from build123d import *

# Parameters (mm, degrees)
SKETCH001_R      = 5
EXTRUDE001_DEPTH = 4
SKETCH_R         = 12.3
EXTRUDE_DEPTH    = 5
BOX001_W         = 82
BOX001_H         = 58
BOX001_DEPTH     = 44.4
BOX_W            = 74.7
BOX_H            = 38.74
BOX_DEPTH        = 44.4


with BuildPart() as extrude001:
    # Sketch001 (on Face3 of Extrude) → Extrude001 (new body)
    with BuildSketch(Plane.XY.offset(49.4)):
        with Locations((-58.7, 20.37)):
            Circle(SKETCH001_R)
    extrude(amount=EXTRUDE001_DEPTH)


with BuildPart() as extrude_body:
    # Sketch (on Face6 of Box001) → Extrude (new body)
    with BuildSketch(Plane(origin=(-82, -9.63, 44.4), x_dir=(1, 0, 0), z_dir=(0, 0, 1))):
        with Locations((23.3, 30)):
            Circle(SKETCH_R)
    extrude(amount=EXTRUDE_DEPTH)


with BuildPart() as cube001:
    # Box001 → Box001 (new body)
    with BuildSketch(Plane(origin=(-82, -9.63, 0), x_dir=(1, 0, 0), z_dir=(0, 0, 1))):
        with Locations((41, 29)):
            Rectangle(BOX001_W, BOX001_H)
    extrude(amount=BOX001_DEPTH)


with BuildPart() as fusion003:
    # Box → Box (new body)
    with BuildSketch(Plane.XY):
        with Locations((37.35, 19.37)):
            Rectangle(BOX_W, BOX_H)
    extrude(amount=BOX_DEPTH)

    # Fusion: union Cube001
    add(cube001.part)

    # Fusion002: union Extrude body
    add(extrude_body.part)

    # Fusion003: union Extrude001
    add(extrude001.part)


solid = fusion003.part
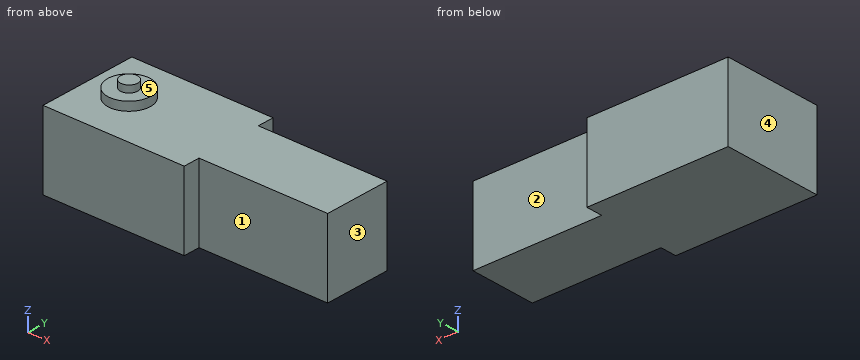
For this review, take the finished solid that the model builds, in its own axes (mm). Face numbers are marked on the shaded views. A direction names the side the tool comes from. Give positions to 0.01 mm unless a question says otherwise; leave off trailing zeros. Loops run counter-clockwise (first coordinate to the right, second up) from the corner with the lowest first, then second, coordinate; pieces in that order, holes last. Notation, with made-up numbers: M 38.5,73 L 89.5,73 A24 cw 89.5,87 Z; hole C 14.5,37.5 d2. An arc over 180 degrees is marked long. Answer as a JSON object with one key per item and string values. Group by question number.
Q1. Tool access review of the marked faces 1, 2, 3, 4 and 5: name each direction out of +Z, -Z, +X, -X, +Y, -Y from which nothing blocks a thin tool from reaching the whole face with its end or side.
Q2. Insertion check: P1, Ø17.5, axis at x = -10, y = 22.5, coming from the +Z side; P2, Ø8, axis at x = 49.5, z = 21, coming from the +Y side; P3, Ø1, axis at x = 18, z = 9.5, coming from the -Y side. Each pin has a flat end and moves straight along its axis. Give the tip position at first contact, or say it passes through.
Q3. Add section B-B on y = 20.37. Give the boundary of the cut face in (x, z).
Q4. Add section C-C on z = 4. Give the boundary of the cut face in (x, y), and give its area (3 significant figures).
Q5. For probe 1 along Z at (x, y) = (42, 30); probe 2 along Y at (x, z) = (28, 7); probe 3 along X at (y, z) = (-2.5, 40.5), list the stretches that pass through material, from the lowest coordinate up. Write a range as [from, to].
Q6. Add section D-D on x = -13. Give the boundary of the cut face in (y, z), and give its area (3 significant figures).
Q7. Add section A-A on x = -58.7. Give the boundary of the cut face in (y, z), and give its area (3 significant figures).
Checked values:
{
 "1": {"face 1": "+Z, -Z, +X, -Y", "face 2": "+Z, -Z, +X, +Y", "face 3": "+Z, -Z, +X, +Y, -Y", "face 4": "+Z, -Z, -X, +Y, -Y", "face 5": "+Z"},
 "2": {"P1": "z = 44.4", "P2": "y = 38.74", "P3": "y = 0"},
 "3": {"outline": "M -82,0 L 74.7,0 L 74.7,44.4 L -46.4,44.4 L -46.4,49.4 L -53.7,49.4 L -53.7,53.4 L -63.7,53.4 L -63.7,49.4 L -71,49.4 L -71,44.4 L -82,44.4 Z"},
 "4": {"outline": "M -82,-9.63 L 0,-9.63 L 0,0 L 74.7,0 L 74.7,38.74 L 0,38.74 L 0,48.37 L -82,48.37 Z", "area": "7,650 mm²"},
 "5": {"probe 1": "[0, 44.4]", "probe 2": "[0, 38.74]", "probe 3": "[-82, 0]"},
 "6": {"outline": "M -9.63,0 L 48.37,0 L 48.37,44.4 L -9.63,44.4 Z", "area": "2,580 mm²"},
 "7": {"outline": "M -9.63,0 L 48.37,0 L 48.37,44.4 L 32.67,44.4 L 32.67,49.4 L 25.37,49.4 L 25.37,53.4 L 15.37,53.4 L 15.37,49.4 L 8.07,49.4 L 8.07,44.4 L -9.63,44.4 Z", "area": "2,740 mm²"}
}
